Source: CAD feature listing. Evaluate the final solid. Frame: model axes, mm. Face numbers are marked on the shaded views. A direction names the side the tool comes from. Give positions to 0.01 mm unless a question says otherwise; leave off trailing zeros. Order: outer loops, then holes, each group sorted by start corner. A loop starts at its lowest first (then second) coordinate and runs counter-clockwise, first axis right, second up.
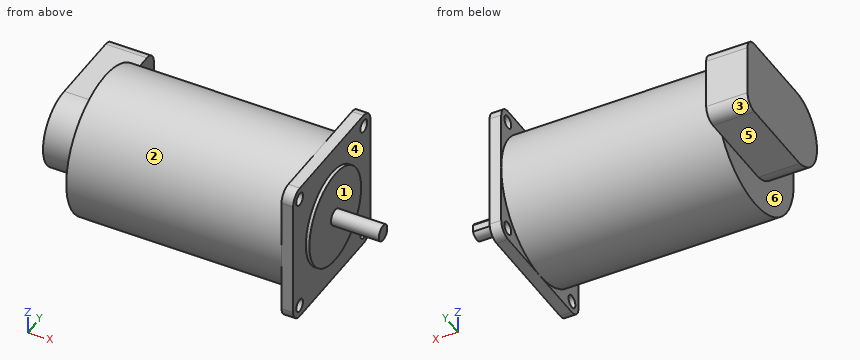
from build123d import *

# Parameters (mm, degrees)
SKETCH1_R           = 28.35
BOSS_EXTRUDE1_DEPTH = 85.4
SKETCH2_W           = 56.7
SKETCH2_H           = 56.7
SKETCH2_R           = 2.5
BOSS_EXTRUDE2_DEPTH = 4.6
SKETCH3_R           = 19
BOSS_EXTRUDE3_DEPTH = 1.4
BOSS_EXTRUDE4_DEPTH = 19
FILLET1_R           = 5
BOSS_EXTRUDE5_DEPTH = 16.4


with BuildPart() as part:
    # Sketch1 → Boss-Extrude1 (new body)
    with BuildSketch(Plane(origin=(0, 0, 0), x_dir=(0, 0, -1), z_dir=(1, 0, 0))):
        with Locations(Location((0, 0, 0), (0, 0, 180))):
            Circle(SKETCH1_R)
    extrude(amount=BOSS_EXTRUDE1_DEPTH)

    # Sketch2 → Boss-Extrude2 (add)
    with BuildSketch(Plane(origin=(85.4, 0, 0), x_dir=(0, 0, -1), z_dir=(1, 0, 0))):
        Rectangle(SKETCH2_W, SKETCH2_H)
        with Locations((-23.55, 23.55)):
            Circle(SKETCH2_R, mode=Mode.SUBTRACT)
        with Locations((23.55, 23.55)):
            Circle(SKETCH2_R, mode=Mode.SUBTRACT)
        with Locations((23.55, -23.55)):
            Circle(SKETCH2_R, mode=Mode.SUBTRACT)
        with Locations((-23.55, -23.55)):
            Circle(SKETCH2_R, mode=Mode.SUBTRACT)
    extrude(amount=BOSS_EXTRUDE2_DEPTH)

    # Sketch3 → Boss-Extrude3 (add)
    with BuildSketch(Plane(origin=(90, 0, 0), x_dir=(0, 0, -1), z_dir=(1, 0, 0))):
        Circle(SKETCH3_R)
    extrude(amount=BOSS_EXTRUDE3_DEPTH)

    # Sketch4 → Boss-Extrude4 (add)
    with BuildSketch(Plane(origin=(91.4, 0, 0), x_dir=(0, 0, -1), z_dir=(1, 0, 0))):
        with BuildLine():
            Line((-1.449137675, 2.825), (1.449137675, 2.825))
            ThreePointArc((1.449137675, 2.825), (0, -3.175), (-1.449137675, 2.825))
        make_face()
    extrude(amount=BOSS_EXTRUDE4_DEPTH)

    # Fillet1
    fillet1_edges = [part.edges().sort_by_distance(p)[0] for p in [
        (87.7, -28.35, 28.35),
        (87.7, -28.35, -28.35),
        (87.7, 28.35, -28.35),
        (87.7, 28.35, 28.35),
    ]]
    fillet(fillet1_edges, radius=FILLET1_R)

    # Sketch5 → Boss-Extrude5 (add)
    with BuildSketch(Plane.ZY):
        with BuildLine():
            Line((-14.919834855, -2.268447858), (-14.919834855, 30.908700262))
            ThreePointArc((-14.919834855, 30.908700262), (-13.455368761, 34.444234167), (-9.919834855, 35.908700262))
            Line((-9.919834855, 35.908700262), (10.080165145, 35.908700262))
            ThreePointArc((10.080165145, 35.908700262), (13.615699051, 34.444234167), (15.080165145, 30.908700262))
            Line((15.080165145, 30.908700262), (15.080165145, 0.579609357))
            ThreePointArc((15.080165145, 0.579609357), (1.426283256, -15.023749328), (-14.919834855, -2.268447858))
        make_face()
    extrude(amount=BOSS_EXTRUDE5_DEPTH)


solid = part.part
1) Reachability of the marked faces 4, 5 and 6 from +Z, -Z, +X, -X, +Y, -Y: full face, straight path, thin tool, end or side. Return the list, or none.
Checks:
face 4: +X
face 5: -Z, -X, +Y, -Y
face 6: -X, -Y
2) Section query A-A on y = 8.5. Output: boundary loops of the cut face in (x, z).
Checks:
outline: (-16.4, -14.92) - (0, -14.92) - (0, -27.05) - (85.4, -27.05) - (85.4, -28.35) - (90, -28.35) - (90, -16.99) - (91.4, -16.99) - (91.4, 16.99) - (90, 16.99) - (90, 28.35) - (85.4, 28.35) - (85.4, 27.05) - (0, 27.05) - (0, 15.08) - (-16.4, 15.08) - close
3) Section query B-B on x = 70. Output: boundary loops of the cut face in (y, z).
Checks:
outline: circle Ø56.7 at (0, 0)
4) Ray query, L1, parallel to Y at x = 86.9, z = 23.55; L2, parallel to Y at x = 86, z = 23. Return the intervals inside material, ascending.
Checks:
L1: y = -28.35 to -26.05, -21.05 to 21.05, 26.05 to 28.35
L2: y = -28.35 to -25.99, -21.11 to 21.11, 25.99 to 28.35
5) First-contact query: pin 1 Ø4 at (y, z) = (23.55, -23.55) entering from -X; pin 2 Ø5 at (x, y) = (-4.5, 13.5) entering from -Z; pin 3 Ø2.5 at (x, z) = (101, 0) entering from +Y (3 decimals); pin 4 Ø8 at (x, y) = (-12, 10) entering from +Z. Flat tips, straight axial feed; report the tip coordinate or a pass-through.
Checks:
pin 1: passes through
pin 2: stops at z = -14.92
pin 3: stops at y = 2.825
pin 4: stops at z = 15.08
6) Pull-direction query (X, two-part tool) for the marked faces 1, 2 and 3; classes: +X half, -X half, draft (parallel to the pull), parting line (faces both ways), or undercut.
Checks:
face 1: +X half
face 2: undercut
face 3: draft
